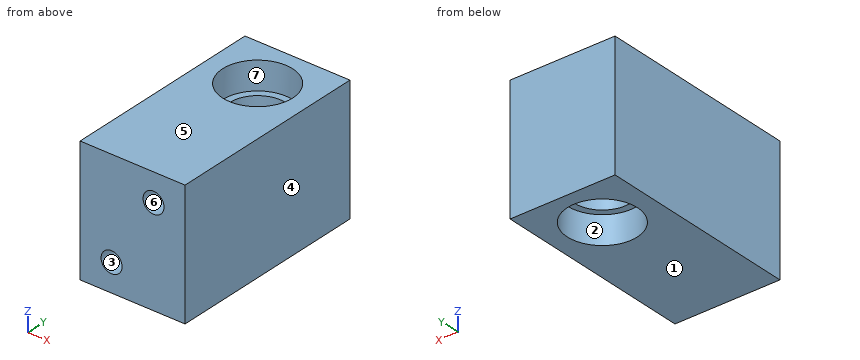
```python
from build123d import *

# Parameters (mm, degrees)
CYLINDER095_R      = 1.5
CYLINDER095_DEPTH  = 21
CYLINDER094_R      = 1.5
CYLINDER094_DEPTH  = 21
CYLINDER085_R      = 4
CYLINDER085_DEPTH  = 19
CYLINDER087_R      = 5
CYLINDER087_DEPTH  = 4
CYLINDER086_R      = 5
CYLINDER086_DEPTH  = 4
BOX406008013_W     = 15
BOX406008013_H     = 29
BOX406008013_DEPTH = 18


with BuildPart() as cylinder095:
    # Cylinder095 → Cylinder095 (new body)
    with BuildSketch(Plane(origin=(3, -13, -4), x_dir=(1, 0, 0), z_dir=(0, -1, 0))):
        Circle(CYLINDER095_R)
    extrude(amount=CYLINDER095_DEPTH)


with BuildPart() as fusion103077013004017014:
    # Cylinder094 → Cylinder094 (new body)
    with BuildSketch(Plane(origin=(-3, -13, -14), x_dir=(1, 0, 0), z_dir=(0, -1, 0))):
        Circle(CYLINDER094_R)
    extrude(amount=CYLINDER094_DEPTH)

    # Fusion103077013004017014: union Cylinder095
    add(cylinder095.part)


with BuildPart() as cylinder081:
    # Cylinder085 → Cylinder085 (new body)
    with BuildSketch(Plane.XY.offset(-17)):
        Circle(CYLINDER085_R)
    extrude(amount=CYLINDER085_DEPTH)


with BuildPart() as f_623_bearing003:
    # Cylinder087 → Cylinder087 (new body)
    with BuildSketch(Plane.XY.offset(-18)):
        Circle(CYLINDER087_R)
    extrude(amount=CYLINDER087_DEPTH)


with BuildPart() as f_623_bearing_holes:
    # Cylinder086 → Cylinder086 (new body)
    with BuildSketch(Plane.XY.offset(-4)):
        Circle(CYLINDER086_R)
    extrude(amount=CYLINDER086_DEPTH)

    # Fusion103077013004017008: union 623 Bearing003
    add(f_623_bearing003.part)


with BuildPart() as cut088:
    # Box406008013 → Box406008013 (new body)
    with BuildSketch(Plane(origin=(-7.5, -22, -18), x_dir=(1, 0, 0), z_dir=(0, 0, 1))):
        with Locations((7.5, 14.5)):
            Rectangle(BOX406008013_W, BOX406008013_H)
    extrude(amount=BOX406008013_DEPTH)

    # Cut070: cut 623 Bearing Holes
    add(f_623_bearing_holes.part, mode=Mode.SUBTRACT)

    # Cut087: cut Cylinder081
    add(cylinder081.part, mode=Mode.SUBTRACT)

    # Cut088: cut Fusion103077013004017014
    add(fusion103077013004017014.part, mode=Mode.SUBTRACT)


solid = cut088.part
```
Input: part model. Units: mm. Frame: model coordinates. Face numbers are marked on the shaded views. A direction names the side the tool comes from. Round coordinates to 2 decimals unless told otherwise and drop trailing zeros. Loops run counter-clockwise (first coordinate to the right, second up) from the corner with the lowest first, then second, coordinate; pieces in that order, holes last. Notation, with made-up numbers: (-5, 87.5) -> (34, 87.5) arc R13 cw to (34, 108.5) -> close; hole circle Ø10 at (21, -20). An arc over 180 degrees is marked (long way). Write each question's results on one line, items separated by ' | '.
1. Section A-A (y = 0). Return loops of the section in (x, z), and give its area (3 significant figures).
Geometry results:
outline: (-7.5, -18) -> (-5, -18) -> (-5, -14) -> (-4, -14) -> (-4, -4) -> (-5, -4) -> (-5, 0) -> (-7.5, 0) -> close; (4, -14) -> (5, -14) -> (5, -18) -> (7.5, -18) -> (7.5, 0) -> (5, 0) -> (5, -4) -> (4, -4) -> close | area: 110 mm2
2. Section C-C (z = -10). Return loops of the section in (x, y), and give its area (3 significant figures).
Geometry results:
outline: (-7.5, -22) -> (7.5, -22) -> (7.5, 7) -> (-7.5, 7) -> close; hole circle Ø8 at (0, 0) | area: 385 mm2
3. Mould query, pull axis X, two halves, no side actions, for the marked faces 1, 2, 3 and 4. Classes: +X half, -X half, draft (parallel to the pull), parting line (faces both ways), or undercut.
Geometry results:
face 1: draft | face 2: undercut | face 3: undercut | face 4: +X half
4. Section B-B (x = 0). Return loops of the section in (y, z), and give its area (3 significant figures).
Geometry results:
outline: (-22, -18) -> (-5, -18) -> (-5, -14) -> (-4, -14) -> (-4, -4) -> (-5, -4) -> (-5, 0) -> (-22, 0) -> close; (4, -14) -> (5, -14) -> (5, -18) -> (7, -18) -> (7, 0) -> (5, 0) -> (5, -4) -> (4, -4) -> close | area: 362 mm2
5. Section D-D (z = -2). Return loops of the section in (x, y), and give its area (3 significant figures).
Geometry results:
outline: (-7.5, -22) -> (7.5, -22) -> (7.5, 7) -> (-7.5, 7) -> close; hole circle Ø10 at (0, 0) | area: 356 mm2
6. Ray query, line 1 (Y direction, x = 0, z = -3); line 2 (X direction, y = -17.5, z = -14); line 3 (X direction, y = -18.5, z = -4). Return the intervals inside material, ascending. Write a range as from..to.
Geometry results:
line 1: -22..-5, 5..7 | line 2: -7.5..-4.5, -1.5..7.5 | line 3: -7.5..1.5, 4.5..7.5
7. Set-up query: the marked faces 5, 6 and 7. Return all of +Z, -Z, +X, -X, +Y, -Y with unobstructed straight access to the full face (end or side cutting, diameter ignored); none if empty.
Geometry results:
face 5: +Z, +X, -X, +Y, -Y | face 6: -Y | face 7: +Z
8. First-contact query: P1, Ø1.5, axis at x = 3.5, z = -3.5, coming from the -Y side; P2, Ø9, axis at x = 0, y = 0, coming from the -Z side; P3, Ø5, axis at x = 0, y = 1, coming from the +Z side. Flat tips, straight axial feed; report the tip coordinate or a pass-through.
Geometry results:
P1: y = -13 | P2: z = -14 | P3: through
